Source: CAD feature listing. Evaluate the final solid. Frame: model axes, mm. A direction names the side the tool comes from. Round coordinates to 2 decimals unless told otherwise and drop trailing zeros. Write each loop counter-clockwise with the first axis right and the second up, starting at its lowest first coordinate (ties: lowest second). Pieces come first, ordered by that corner, then holes. Notation, with made-up numbers: M 76,66 L 132,66 A21 cw 132,75 Z; hole C 74,44 d3. An arc over 180 degrees is marked long. Answer in a Markdown table with one row per item. Add a question column.
Item 1: Cut plane A-A on x = 8. Return loops of the section in (y, z).
Item 2: Material intervals for probe 1 along X at (y, z) = (0.6, 7); probe 2 along X at (y, z) = (0.25, 7); probe 3 along Y at (x, z) = (8, 1.45), sorted ascending.
Item 3: Cut plane C-C on z = 7. Return loops of the section in (x, y), and give its area (3 significant figures).
Item 4: Cut plane B-B on y = 2.5. Return loops of the section in (x, z), and give its area (3 significant figures).
Item 5: Mould query, pull axis X, two halves, no side actions, for faces 1 (the face through (15.715, 0.762, 9.699)), 2 (the face through (11, 0, 4)), 3 (the face through (0.285, 4.699, 1.014)), 4 (the face through (15, 0.3, 6)). Classes: released by +X, released by -X, zero draft, split by the parting line, or undercut.
Item 6: Contact query for flat-ended pins moving along their axis: pin 1 (1 mm diameter, centred on y = 3.5, z = 7, fed in from +X); pin 2 (4 mm diameter, centred on x = 13.5, z = 7, fed in from +Y); pin 3 (4.5 mm diameter, centred on x = 3.5, z = 8, fed in from -Y); pin 4 (3 mm diameter, centred on x = 8, y = 2.5, fed in from +Z). Output: stop coordinate, or through.
Item 7: Set-up query: faces 5 (the face through (10.801, 0.762, 9.715)), 6 (the face through (3, 1.504, 5)), 7 (the face through (4, 0.3, 6)). Return all of +Z, -Z, +X, -X, +Y, -Y with unobstructed straight access to the full face (end or side cutting, diameter ignored); none if empty.
Item 8: Cut plane D-D on z = 2.5. Return loops of the section in (x, y).
from build123d import *

# Parameters (mm, degrees)
SKETCH_1_W          = 16
SKETCH_1_H          = 5
EXTRUDE_1_DEPTH     = 10
SKETCH_2_W          = 16
SKETCH_2_H          = 3.496194888
CUT_EXTRUDE_1_DEPTH = 8
SKETCH_4_W          = 5
SKETCH_4_H          = 1.503805112
CUT_EXTRUDE_3_DEPTH = 8
SKETCH_3_R          = 1.3
CUT_EXTRUDE_2_DEPTH = 2
SKETCH_5_R          = 1.5
CUT_EXTRUDE_5_DEPTH = 2
SKETCH_6_R          = 2
CUT_EXTRUDE_6_DEPTH = 0.3
FILLET_1_R          = 1
FILLET_2_R          = 1
CHAMFER_1_SIZE      = 0.5


with BuildPart() as part:
    # 草图1 → 凸台-拉伸1 (new body)
    with BuildSketch(Plane.XY):
        with Locations((8, 2.5)):
            Rectangle(SKETCH_1_W, SKETCH_1_H)
    extrude(amount=EXTRUDE_1_DEPTH)

    # 草图2 → 切除-拉伸1 (cut)
    with BuildSketch(Plane.XY.offset(10)):
        with Locations((8, 3.251902556)):
            Rectangle(SKETCH_2_W, SKETCH_2_H)
    extrude(amount=-CUT_EXTRUDE_1_DEPTH, mode=Mode.SUBTRACT)

    # 草图4 → 切除-拉伸3 (cut)
    with BuildSketch(Plane.XY.offset(10)):
        with Locations((8, 0.751902556)):
            Rectangle(SKETCH_4_W, SKETCH_4_H)
    extrude(amount=-CUT_EXTRUDE_3_DEPTH, mode=Mode.SUBTRACT)

    # 草图3 → 切除-拉伸2 (cut)
    with BuildSketch(Plane.XY.offset(2)):
        with Locations((8, 2.5)):
            Circle(SKETCH_3_R)
    extrude(amount=-CUT_EXTRUDE_2_DEPTH, mode=Mode.SUBTRACT)

    # 草图5 → 切除-拉伸5 (cut)
    with BuildSketch(Plane.XZ):
        with Locations(Location((2.5, 7, 0), (0, 0, 270))):
            Circle(SKETCH_5_R)
        with Locations(Location((13.5, 7, 0), (0, 0, 270))):
            Circle(SKETCH_5_R)
    extrude(amount=-CUT_EXTRUDE_5_DEPTH, mode=Mode.SUBTRACT)

    # 草图6 → 切除-拉伸6 (cut)
    with BuildSketch(Plane.XZ):
        with Locations(Location((2.5, 7, 0), (0, 0, 270))):
            Circle(SKETCH_6_R)
        with Locations(Location((13.5, 7, 0), (0, 0, 270))):
            Circle(SKETCH_6_R)
    extrude(amount=-CUT_EXTRUDE_6_DEPTH, mode=Mode.SUBTRACT)

    # 圆角1
    fillet_1_edges = [part.edges().sort_by_distance(p)[0] for p in [
        (0, 5, 1),
        (16, 5, 1),
    ]]
    fillet(fillet_1_edges, radius=FILLET_1_R)

    # 圆角2
    fillet_2_edges = [part.edges().sort_by_distance(p)[0] for p in [
        (16, 0.751902556, 10),
        (0, 0.751902556, 10),
        (5.5, 0.751902556, 10),
        (10.5, 0.751902556, 10),
    ]]
    fillet(fillet_2_edges, radius=FILLET_2_R)

    # 倒角1
    chamfer_1_edges = [part.edges().sort_by_distance(p)[0] for p in [
        (8, 0, 0),
    ]]
    chamfer(chamfer_1_edges, length=CHAMFER_1_SIZE)


solid = part.part
Results below:
| question | item | result |
|---|---|---|
| 1 | outline | M 0,0.5 L 0.5,0 L 1.2,0 L 1.2,2 L 0,2 Z; M 3.8,0 L 5,0 L 5,2 L 3.8,2 Z |
| 2 | probe 1 | 0 to 1, 4 to 5.5, 10.5 to 12, 15 to 16 |
| 2 | probe 2 | 0 to 0.5, 4.5 to 5.5, 10.5 to 11.5, 15.5 to 16 |
| 2 | probe 3 | 0 to 1.2, 3.8 to 5 |
| 3 | outline | M 0,0 L 0.5,0 L 0.5,0.3 L 1,0.3 L 1,1.5 L 0,1.5 Z; M 4,0.3 L 4.5,0.3 L 4.5,0 L 5.5,0 L 5.5,1.5 L 4,1.5 Z; M 10.5,0 L 11.5,0 L 11.5,0.3 L 12,0.3 L 12,1.5 L 10.5,1.5 Z; M 15,0.3 L 15.5,0.3 L 15.5,0 L 16,0 L 16,1.5 L 15,1.5 Z |
| 3 | area | 6.92 mm2 |
| 4 | outline | M 0,0 L 6.7,0 L 6.7,2 L 0,2 Z; M 9.3,0 L 16,0 L 16,2 L 9.3,2 Z |
| 4 | area | 26.8 mm2 |
| 5 | face 1 | released by +X |
| 5 | face 2 | zero draft |
| 5 | face 3 | released by -X |
| 5 | face 4 | undercut |
| 6 | pin 1 | through |
| 6 | pin 2 | y = 1.5 |
| 6 | pin 3 | y = 0 |
| 6 | pin 4 | z = 2 |
| 7 | face 5 | +Z, +Y, -Y |
| 7 | face 6 | +Z, +X, -X, +Y |
| 7 | face 7 | -Y |
| 8 | outline | M 0,0 L 5.5,0 L 5.5,1.5 L 0,1.5 Z; M 10.5,0 L 16,0 L 16,1.5 L 10.5,1.5 Z |
